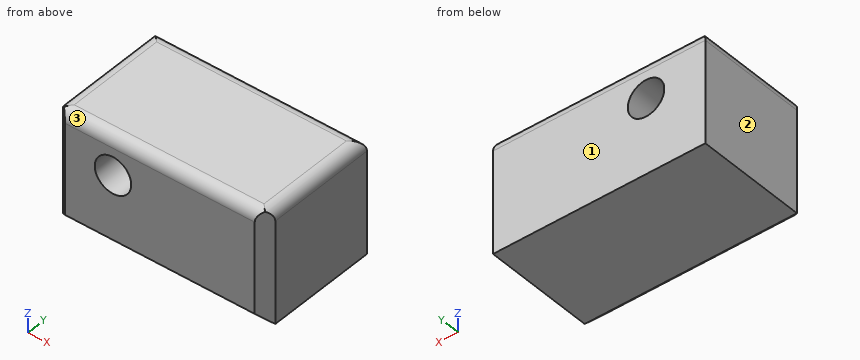
```python
from build123d import *

# Parameters (mm, degrees)
F0_W        = 95.7747641951
F0_H        = 51.2457955629
F1_DEPTH    = 55.118
F2_R        = 5.08
F3_T1_DEPTH = 72.2940947206
F3_T3_DEPTH = 121.9030633528
F4_R        = 8.2354501167
F5_DEPTH    = 129.032


# Not quite as in the source:
# - a fillet or chamfer that OpenCascade refuses, or shapes differently, is made with other operations: its cross-section is extruded or revolved along the edge and cut away or added


with BuildPart() as f1:
    # F0 (on Front) → F1 (new body)
    with BuildSketch(Plane.XZ):
        with Locations((-20.3259242699, 5.727651529)):
            Rectangle(F0_W, F0_H)
    extrude(amount=F1_DEPTH)

    # F2
    f2_edges = [f1.edges().sort_by_distance(p)[0] for p in [
        (27.561458, -27.559, 31.350549),
        (-68.213306, -27.559, 31.350549),
        (-20.325924, 0, 31.350549),
        (-20.325924, -55.118, 31.350549),
    ]]
    fillet(f2_edges, radius=F2_R)

    # F3: chamfer of 5.08 on 4 edges, made by hand

    # F3_s2 → F3_t1 (cut)
    with BuildSketch(Plane.XY.offset(-32.9593958313)):
        Polygon((-63.1333063674, -55.118), (-68.2133063674, -50.038), (-68.2133063674, -55.118), align=None)
        Polygon((27.5614578277, -50.038), (22.4814578277, -55.118), (27.5614578277, -55.118), align=None)
    extrude(amount=F3_T1_DEPTH, mode=Mode.SUBTRACT)

    # F3_s4 → F3_t3 (cut)
    with BuildSketch(Plane.YZ.offset(-81.2774559463)):
        Polygon((-55.118, -14.8152462524), (-50.038, -19.8952462524), (-55.118, -19.8952462524), align=None)
    extrude(amount=F3_T3_DEPTH, mode=Mode.SUBTRACT)

    # F4 (on face) → F5 (cut)
    with BuildSketch(Plane.XZ.offset(55.118)):
        with Locations((-41.4717569947, 14.13862966)):
            Circle(F4_R)
    extrude(amount=-F5_DEPTH, mode=Mode.SUBTRACT)


solid = f1.part
```
Can you work these out from the model? Positions are in its coordinate system, mm. Face numbers are marked on the shaded views. Give positions to 0.01 mm unless a question says otherwise; leave off trailing zeros. Loops run counter-clockwise (first coordinate to the right, second up) from the corner with the lowest first, then second, coordinate; pieces in that order, holes last. Notation, with made-up numbers: M 7.25,27.25 L 41.25,27.25 A25 ccw 41.25,41.25 Z; hole C 11.25,-3.75 d8. An arc over 180 degrees is marked long. Answer in a Markdown table with one row per item.
1. Suppose I cut it at B-B on y = -40. Write out the boundary of the cut face in (x, z).
Taken from the geometry:
| item | result |
|---|---|
| outline | M -68.21,-19.9 L 27.56,-19.9 L 27.56,26.27 A5.08 ccw 22.48,31.35 L -63.13,31.35 A5.08 ccw -68.21,26.27 Z; hole C -41.47,14.14 d16.47 |
2. Thinking about a two-plate mould opening in Y: for the marked faces 1, 2 and 3, which applies, released by +Y, released by -Y, zero draft, split by the parting line, or undercut?
Taken from the geometry:
| item | result |
|---|---|
| face 1 | released by +Y |
| face 2 | zero draft |
| face 3 | released by -Y |
3. For pin 1 Ø4 at (x, z) = (-11.5, 24.5) entering from +Y, with a flat end and sliding along its axis, tell me the tip position at first contact or that it passes through.
Taken from the geometry:
| item | result |
|---|---|
| pin 1 | stops at y = 0 |
4. Suppose I cut it at A-A on x = -39. Write out the boundary of the cut face in (y, z), plus the area to 3 significant figures.
Taken from the geometry:
| item | result |
|---|---|
| outline | M -55.12,-14.82 L -50.04,-19.9 L 0,-19.9 L 0,6.28 L -55.12,6.28 Z; M -55.12,21.99 L 0,21.99 L 0,26.27 A5.08 ccw -5.08,31.35 L -50.04,31.35 A5.08 ccw -55.12,26.27 Z |
| area | 1,930 mm² |
5. Suppose I cut it at D-D on y = -51.5. Write out the boundary of the cut face in (x, z).
Taken from the geometry:
| item | result |
|---|---|
| outline | M -66.75,-18.43 L 26.1,-18.43 L 26.1,29.84 A5.08 ccw 23.94,31.14 L -64.6,31.14 A5.08 ccw -66.75,29.84 Z; hole C -41.47,14.14 d16.47 |
6. Suppose I cut it at C-C on z = 19. Write out the boundary of the cut face in (x, y), plus the area to 3 significant figures.
Taken from the geometry:
| item | result |
|---|---|
| outline | M -68.21,-50.04 L -63.13,-55.12 L -48.12,-55.12 L -48.12,0 L -68.21,0 Z; M -34.82,-55.12 L 22.48,-55.12 L 27.56,-50.04 L 27.56,0 L -34.82,0 Z |
| area | 4,520 mm² |
7. If I drill on line 1 along Z through (x, y) = (22.5, -2.5); line 2 along X through (y, z) = (-5.5, 8); line 3 along Z through (x, y) = (-39.5, -27), over which ranges is the centre line in solid material (lowest first)?
Taken from the geometry:
| item | result |
|---|---|
| line 1 | z = -19.9 to 30.65 |
| line 2 | x = -68.21 to -46.96, -35.98 to 27.56 |
| line 3 | z = -19.9 to 6.14, 22.13 to 31.35 |
